Read the model definition and answer for the solid it produces. Units are mm, in the model's axes. Round coordinates to 2 decimals unless told otherwise and drop trailing zeros. Order: outer loops, then holes, each group sorted by start corner. A loop starts at its lowest first (then second) coordinate and runs counter-clockwise, first axis right, second up. Notation, with made-up numbers: (-11, 5) -> (39, 5) arc R25 cw to (39, 26) -> close; hole circle Ø5 at (28.5, 79). An arc over 180 degrees is marked (long way). One line per item, written item: value. Start each with the question number.
1. Section C-C (y = 1.75) is taken. Give the vertices of the cut face in (x, z), then the cut area to 3 significant figures.
2. Section B-B (x = 47) is taken. Give the vertices of the cut face in (y, z).
3. Section A-A (z = 0) is taken. Give the vertices of the cut face in (x, y), then the cut area to 4 significant figures.
4. Flat-ended cylindrical pins translate along their axes: pin 1 Ø1.5 at (y, z) = (2, -6) entering from -X; pin 2 Ø1 at (x, y) = (45, 2) entering from -Z. Find the tip coordinate at first contact, or state that the pin passes through.
5. Consider line 1 (X direction, y = 1.35, z = 1); line 2 (X direction, y = 0.9, z = -0.5); line 3 (X direction, y = 0.45, z = -2.5). Determine where each line is inside the solid, lowest interval first.
6. Section D-D (x = 39.5) is taken. Give the vertices of the cut face in (y, z).
from build123d import *

# Parameters (mm, degrees)
BOSS_EXTRUDE1_DEPTH = 3
CUT_EXTRUDE1_REACH  = 55.528
SKETCH2_R           = 1.5
SKETCH2_R_2         = 4


with BuildPart() as part:
    # Sketch1 → Boss-Extrude1 (new body)
    with BuildSketch(Plane(origin=(0, 0, 0), x_dir=(1, 0, 0), z_dir=(0, 1, 0))):
        with BuildLine():
            ThreePointArc((0, 10), (-10, 0), (0, -10))
            Line((0, -10), (45.414124006, -7.488558026))
            ThreePointArc((45.414124006, -7.488558026), (52.5, 0), (45.414124006, 7.488558026))
            Line((45.414124006, 7.488558026), (0, 10))
        make_face()
    extrude(amount=BOSS_EXTRUDE1_DEPTH)

    # Sketch2 → Cut-Extrude1 (cut, up to next)
    with BuildSketch(Plane(origin=(0, 3, 0), x_dir=(1, 0, 0), z_dir=(0, 1, 0)), mode=Mode.PRIVATE) as cut_extrude1_sk1:
        with Locations(Location((0, 0, 0), (0, 0, 270))):
            Circle(SKETCH2_R)
    cut_extrude1_tool1 = extrude(cut_extrude1_sk1.sketch, amount=-CUT_EXTRUDE1_REACH, mode=Mode.PRIVATE) & part.part
    # Sketch2 → Cut-Extrude1 (cut, up to next)
    with BuildSketch(Plane(origin=(0, 3, 0), x_dir=(1, 0, 0), z_dir=(0, 1, 0)), mode=Mode.PRIVATE) as cut_extrude1_sk2:
        with Locations(Location((45, 0, 0), (0, 0, 270))):
            Circle(SKETCH2_R_2)
    cut_extrude1_tool2 = extrude(cut_extrude1_sk2.sketch, amount=-CUT_EXTRUDE1_REACH, mode=Mode.PRIVATE) & part.part
    add(cut_extrude1_tool1.solids().sort_by_distance((0, 3, 0))[0], mode=Mode.SUBTRACT)
    add(cut_extrude1_tool2.solids().sort_by_distance((45, 3, 0))[0], mode=Mode.SUBTRACT)


solid = part.part
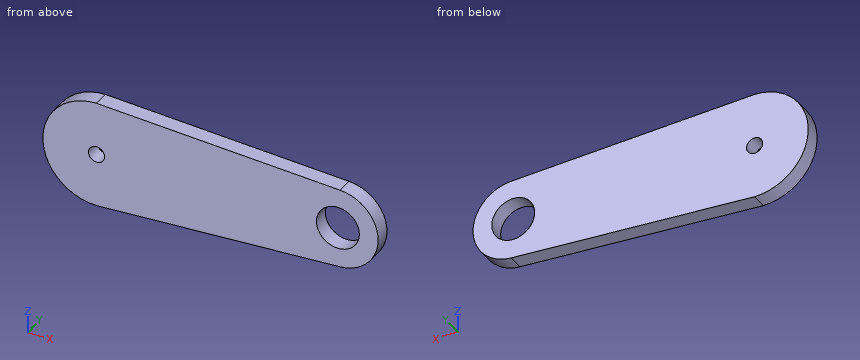
Answer:
1. outline: (0, -10) -> (45.41, -7.49) arc R7.5 ccw to (45.41, 7.49) -> (0, 10) arc R10 ccw to start; hole circle Ø3 at (0, 0); hole circle Ø8 at (45, 0)
1. area: 976 mm^2
2. outline: (0, -7.23) -> (3, -7.23) -> (3, -3.46) -> (0, -3.46) -> close; (0, 3.46) -> (3, 3.46) -> (3, 7.23) -> (0, 7.23) -> close
3. outline: (-10, 0) -> (-1.5, 0) -> (-1.5, 3) -> (-10, 3) -> close; (1.5, 0) -> (41, 0) -> (41, 3) -> (1.5, 3) -> close; (49, 0) -> (52.5, 0) -> (52.5, 3) -> (49, 3) -> close
3. area: 154.5 mm^2
4. pin 1: x = -8.51
4. pin 2: z = -7.54
5. line 1: -9.95 to -1.12, 1.12 to 41.13, 48.87 to 52.43
5. line 2: -9.99 to -1.41, 1.41 to 41.03, 48.97 to 52.48
5. line 3: -9.68 to 41.88, 48.12 to 52.07
6. outline: (0, -7.82) -> (3, -7.82) -> (3, 7.82) -> (0, 7.82) -> close
